Input: part model. Units: mm. Frame: model coordinates. Give positions to 0.01 mm unless a question says otherwise; leave off trailing zeros. Order: outer loops, then holes, each group sorted by start corner. A loop starts at its lowest first (then second) coordinate and runs counter-clockwise, first axis right, second up. Notation, with made-up numbers: (13, -30) - (42, -30) arc R35 ccw to (42, 8) - close; hole circle Ø6 at (67, 72). An arc over 180 degrees is marked (long way). Use a Markdown table: item, result.
from build123d import *

# Parameters (mm, degrees)
BOSS_EXTRU_1_DEPTH      = 20
CONG_1_R                = 3
ESQUISSE2_R             = 1
ENL_V_MAT_EXTRU_1_DEPTH = 10


with BuildPart() as part:
    # Esquisse1 → Boss.-Extru.1 (new body)
    with BuildSketch(Plane.XY):
        Polygon((0, 0), (60, 0), (60, 40), (0, 20), align=None)
    extrude(amount=BOSS_EXTRU_1_DEPTH)

    # Congé1
    cong_1_edges = [part.edges().sort_by_distance(p)[0] for p in [
        (0, 20, 10),
        (60, 40, 10),
        (60, 0, 10),
        (0, 0, 10),
    ]]
    fillet(cong_1_edges, radius=CONG_1_R)

    # Esquisse2 → Enlèv. mat.-Extru.1 (cut)
    with BuildSketch(Plane(origin=(60, 0, 0), x_dir=(0, 0, -1), z_dir=(1, 0, 0))):
        with Locations((-10, 24)):
            Circle(ESQUISSE2_R)
    extrude(amount=-ENL_V_MAT_EXTRU_1_DEPTH, mode=Mode.SUBTRACT)


solid = part.part
1. Section query C-C (x = 39). Return loops of the section in (y, z).
Response:
| item | result |
|---|---|
| outline | (0, 0) - (33, 0) - (33, 20) - (0, 20) - close |
2. Material intervals for line 1 along Y through (x, z) = (52.5, 10); line 2 along Y through (x, z) = (46, 5.5); line 3 along Y through (x, z) = (36.5, 4), sorted ascending.
Response:
| item | result |
|---|---|
| line 1 | y = 0 to 23, 25 to 37.5 |
| line 2 | y = 0 to 35.33 |
| line 3 | y = 0 to 32.17 |
3. Section query D-D (z = 18). Return loops of the section in (x, y).
Response:
| item | result |
|---|---|
| outline | (0, 3) arc R3 ccw to (3, 0) - (57, 0) arc R3 ccw to (60, 3) - (60, 35.84) arc R3 ccw to (56.05, 38.68) - (2.05, 20.68) arc R3 ccw to (0, 17.84) - close |
4. Mould query, pull axis Z, two halves, no side actions, for faces 1 (the face through (55, 23, 10)), 2 (the face through (50, 24, 10)), 3 (the face through (30, 15, 20)), 4 (the face through (0.58, 19.61, 10.14)). Classes: pulls with the +Z half, pulls with the -Z half, needs draft (parallel to the pull), parting line crosses it, or undercut.
Response:
| item | result |
|---|---|
| face 1 | undercut |
| face 2 | undercut |
| face 3 | pulls with the +Z half |
| face 4 | needs draft |
5. Section query A-A (z = 10). Return loops of the section in (x, y), then the cut area to 3 significant figures.
Response:
| item | result |
|---|---|
| outline | (0, 3) arc R3 ccw to (3, 0) - (57, 0) arc R3 ccw to (60, 3) - (60, 23) - (50, 23) - (50, 25) - (60, 25) - (60, 35.84) arc R3 ccw to (56.05, 38.68) - (2.05, 20.68) arc R3 ccw to (0, 17.84) - close |
| area | 1,770 mm^2 |
6. Pin query (flat end, axial travel): pin 1 (2 mm diameter, centred on x = 17, z = 12.5, fed in from +Y); pin 2 (1.5 mm diameter, centred on x = 6.5, z = 8, fed in from +Y); pin 3 (1.6 mm diameter, centred on y = 24, z = 10, fed in from +X). Return the tip coordinate at first contact, or that it passes through.
Response:
| item | result |
|---|---|
| pin 1 | stops at y = 26 |
| pin 2 | stops at y = 22.42 |
| pin 3 | stops at x = 50 |
7. Section query B-B (y = 24). Return loops of the section in (x, z), then the cut area to 3 significant figures.
Response:
| item | result |
|---|---|
| outline | (12, 0) - (60, 0) - (60, 9) - (50, 9) - (50, 11) - (60, 11) - (60, 20) - (12, 20) - close |
| area | 940 mm^2 |
